CAD build for the part. Positions are in the model's coordinates, mm. A direction names the side the tool comes from. Give positions to 0.01 mm unless a question says otherwise; leave off trailing zeros. Loops run counter-clockwise (first coordinate to the right, second up) from the corner with the lowest first, then second, coordinate; pieces in that order, holes last.
Item 1: Mould opens along Z. For faces 4 (the cylindrical face through (1.97, -5.34, -11.77)), 5 (the cylindrical face through (1.972, 11.774, -5.266)), 6 (the cylindrical face through (1.97, 5.34, 11.77)) say: released by +Z, released by -Z, zero draft, split by the parting line, or undercut.
Item 2: Probe probe 1 along Y at (x, z) = (0.8, 0); probe 2 along Y at (x, z) = (0.5, -11.5); probe 3 along X at (y, z) = (3.25, 1.75). List the from-to ranges inside material, lowest first.
Item 3: Saw through at A-A on y = 8. Give the cut face in (x, z).
Item 4: Drop flat-ended pins along their axis: P1, Ø1, axis at x = -2.5, z = -4.5, coming from the +Y side; P2, Ø3.5, axis at x = -2, y = -1, coming from the -Z side; P3, Ø0.9, axis at x = -2, y = -0.5, coming from the +Z side. Give the stop position or say it passes through.
Item 5: Which spindle directions (+Z, -Z, +X, -X, +Y, -Y) get a long thin tool onto all of the face, cutting with end or side? Do faces 1 (the cylindrical face through (1.97, -12.9, 0.82)), 2 (the cylindrical face through (1.972, 11.023, 6.698)), 3 (the flat face through (-2.521, 5.394, -3.057)). Say none if no direction does.
from build123d import *

# Parameters (mm, degrees)
BASPROSKE_W         = 4
BASPROSKE_H         = 14
TOOTHCUT_DEPTH      = 21.199009877
TEETHCUTS_COUNT     = 26
TEETHCUTS_ANGLE     = 346.153846154
BORSKE_R            = 2
BORE_DEPTH          = 50.0000508
SKETCH_1_R          = 9
SKETCH_1_R_2        = 2
EXTRUDE_1_DEPTH     = 4
CUT_EXTRUDE_1_DEPTH = 3
SKETCH_4_R          = 2.1
CUT_EXTRUDE_2_DEPTH = 22.307778916


with BuildPart() as part:
    # BasProSke → Base-Revolve (revolve)
    with BuildSketch(Plane(origin=(0, 0, 0), x_dir=(1, 0, 0), z_dir=(0, 1, 0)), mode=Mode.PRIVATE) as base_revolve_sk:
        with Locations((2, 7)):
            Rectangle(BASPROSKE_W, BASPROSKE_H)
    revolve(base_revolve_sk.sketch.rotate(Axis((-10, 0, 0), (1, 0, 0)), 180), axis=Axis((-10, 0, 0), (1, 0, 0)))

    # TooCutSke → ToothCut (cut, through all)
    with BuildSketch(Plane(origin=(0, 0, 0), x_dir=(0, 0, -1), z_dir=(1, 0, 0))):
        with BuildLine():
            ThreePointArc((0.476965065, 11.739314517), (0, 11.749), (-0.476965065, 11.739314517))
            ThreePointArc((-0.476965065, 11.739314517), (-0.82065865, 12.901686978), (-1.424117301, 13.952911348))
            ThreePointArc((-1.424117301, 13.952911348), (0, 14.0254), (1.424117301, 13.952911348))
            ThreePointArc((1.424117301, 13.952911348), (0.82065865, 12.901686978), (0.476965065, 11.739314517))
        make_face()
    toothcut = extrude(amount=TOOTHCUT_DEPTH, mode=Mode.SUBTRACT)

    # TeethCuts: ToothCut ×26 about axis
    teethcuts_axis = Axis((-10, 0, 0), (1, 0, 0))
    for i in range(1, TEETHCUTS_COUNT):
        add(toothcut.rotate(teethcuts_axis, i * TEETHCUTS_ANGLE / (TEETHCUTS_COUNT - 1)), mode=Mode.SUBTRACT)

    # BorSke → Bore (cut, symmetric)
    with BuildSketch(Plane(origin=(0, 0, 0), x_dir=(0, 0, -1), z_dir=(1, 0, 0))):
        with Locations(Location((0, 0, 0), (0, 0, 180))):
            Circle(BORSKE_R)
    extrude(amount=BORE_DEPTH, both=True, mode=Mode.SUBTRACT)

    # 草图1 → 凸台-拉伸1 (add)
    with BuildSketch(Plane.ZY):
        with Locations(Location((0, 0, 0), (0, 0, 180))):
            Circle(SKETCH_1_R)
        Circle(SKETCH_1_R_2, mode=Mode.SUBTRACT)
    extrude(amount=EXTRUDE_1_DEPTH)

    # 草图2 → 切除-拉伸1 (cut)
    with BuildSketch(Plane.ZY.offset(4)):
        Polygon((6.2, 3.579571669), (0, 7.159143338), (-6.2, 3.579571669), (-6.2, -3.579571669), (0, -7.159143338), (6.2, -3.579571669), align=None)
    extrude(amount=-CUT_EXTRUDE_1_DEPTH, mode=Mode.SUBTRACT)

    # 草图4 → 切除-拉伸2 (cut, through all)
    with BuildSketch(Plane(origin=(4, 0, 0), x_dir=(0, 0, -1), z_dir=(1, 0, 0))):
        Circle(SKETCH_4_R)
    extrude(amount=-CUT_EXTRUDE_2_DEPTH, mode=Mode.SUBTRACT)


solid = part.part
Results below:
1. face 4: released by -Z
1. face 5: undercut
1. face 6: released by +Z
2. probe 1: y = -11.75 to -2.1, 2.1 to 11.75
2. probe 2: y = -6.72 to -5.1, -3.77 to 3.77, 5.1 to 6.72
2. probe 3: x = -1 to 4
3. outline: (-4, -4.12) - (0, -4.12) - (0, -10.15) - (4, -10.15) - (4, 10.15) - (0, 10.15) - (0, 4.12) - (-4, 4.12) - close
4. P1: stops at y = 8.06
4. P2: stops at z = -9
4. P3: stops at z = 9
5. face 1: +X, -X, -Y
5. face 2: +X, -X, +Y
5. face 3: -X
